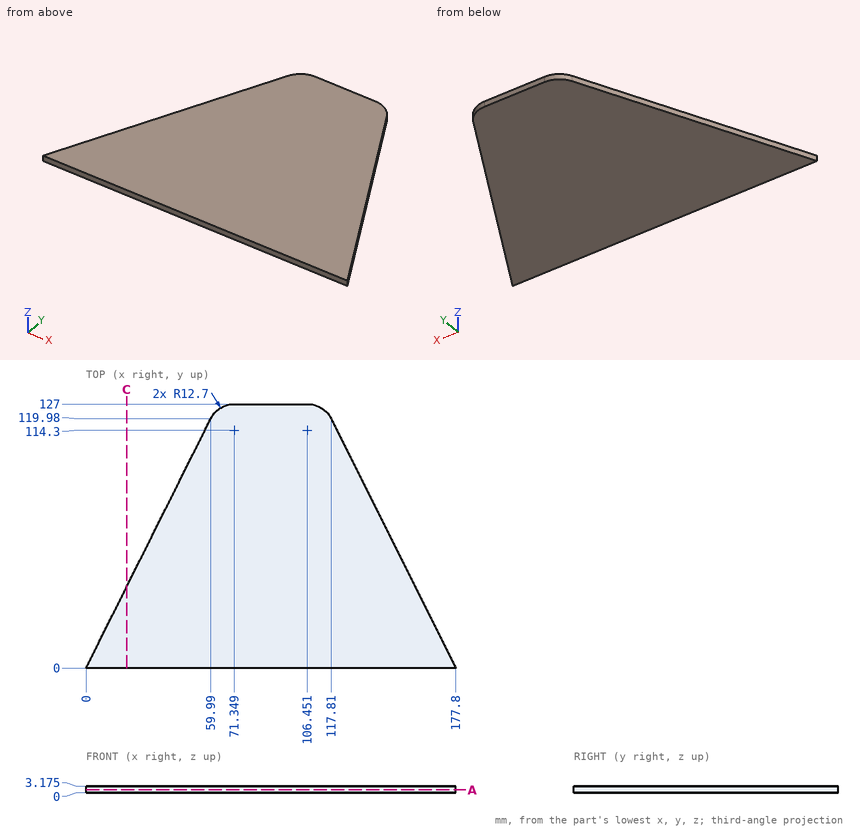
Input: dimensioned drawing with shaded views. Units: mm. Origin: part minimum x, y, z. Give positions to 0.01 mm unless a question says otherwise; leave off trailing zeros. Write each loop counter-clockwise with the first axis right and the second up, starting at its lowest first coordinate (ties: lowest second). Pieces come first, ordered by that corner, then holes. Notation, with made-up numbers: (-6.75, 67.25) - (37.25, 67.25) arc R7 cw to (37.25, 79.25) - close; hole circle Ø2 at (-14.75, 6). An arc over 180 degrees is marked (long way). Write item = value, one per line. Start each with the question number.
1) Material intervals for L1, parallel to X at y = 34, z = 2.1; L2, parallel to X at y = 49, z = 2.9; L3, parallel to Y at x = 150, z = 1.25, sorted ascending. Write a range as [from, to].
2) Cut plane C-C (x = 19.5). Return loops of the section in (y, z) (1 decimal), and give its area (3 significant figures).
3) Cut plane A-A (z = 1.35). Return loops of the section in (x, y).
4) Pin query (flat end, axial travel): pin 1 (1 mm diameter, centred on y = 54, z = 2, fed in from -X); pin 2 (1 mm diameter, centred on y = 29, z = 1.5, fed in from +X); pin 3 (1.5 mm diameter, centred on x = 60.5, z = 0.5, fed in from +Y); pin 4 (4 mm diameter, centred on x = 151, y = 58, fed in from -Z). Return the tip coordinate at first contact, or that it passes through.
Answers follow:
q1.L1 = [17, 160.8]
q1.L2 = [24.5, 153.3]
q1.L3 = [0, 55.6]
q2.outline = (0, 0) - (39, 0) - (39, 3.2) - (0, 3.2) - close
q2.area = 124 mm^2
q3.outline = (0, 0) - (177.8, 0) - (117.81, 119.98) arc R12.7 ccw to (106.45, 127) - (71.35, 127) arc R12.7 ccw to (59.99, 119.98) - close
q4.pin_1 = 26.75
q4.pin_2 = 163.55
q4.pin_3 = 122
q4.pin_4 = 0
